Input: part model. Units: mm. Frame: model coordinates. Face numbers are marked on the shaded views. Coordinates: 2 decimals unless noted, no trailing zeros. Loops run counter-clockwise (first coordinate to the right, second up) from the corner with the lowest first, then second, coordinate; pieces in that order, holes last. Notation, with made-up numbers: (70, -38) -> (85, -38) arc R22 ccw to (85, -26) -> close; hole circle Ø2 at (84, -1.5). An arc over 180 degrees is marked (long way). Answer as a JSON object with one key per item and string values.
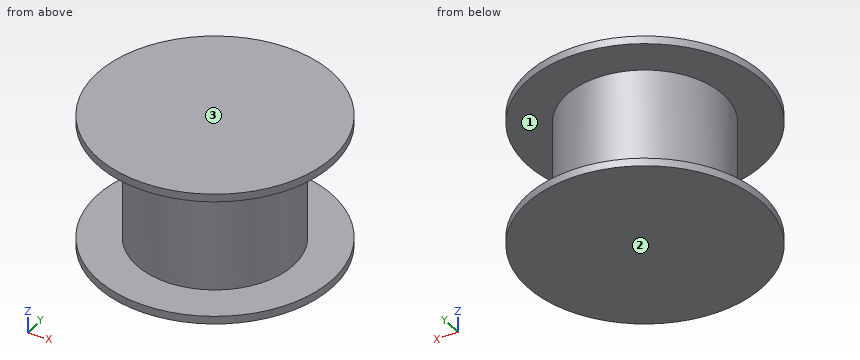
from build123d import *

# Parameters (mm, degrees)
SKETCH1_R           = 10
BOSS_EXTRUDE1_DEPTH = 16
SKETCH2_R           = 15
BOSS_EXTRUDE2_DEPTH = 1
SCALE1_SCALE        = 0.2
SCALE2_SCALE        = 2


with BuildPart() as part:
    # Sketch1 → Boss-Extrude1 (new body)
    with BuildSketch(Plane.XY):
        Circle(SKETCH1_R)
    extrude(amount=BOSS_EXTRUDE1_DEPTH)

    # Sketch2 → Boss-Extrude2 (add)
    with BuildSketch(Plane.XY.offset(16)):
        Circle(SKETCH2_R)
    boss_extrude2 = extrude(amount=-BOSS_EXTRUDE2_DEPTH)

    # Mirror1: Boss-Extrude2 across plane
    add(boss_extrude2.mirror(Plane(origin=(0, 0, 7.5), x_dir=(1, 0, 0), z_dir=(0, 0, -1))))


with BuildPart() as part_1:
    # Scale1: scaled about (0, 0, 7.5)
    add(part.part.scale(SCALE1_SCALE).moved(Location((0, 0, 6))))


with BuildPart() as part_2:
    # Scale2: scaled about (0, 0, 7.5)
    add(part_1.part.scale(SCALE2_SCALE).moved(Location((0, 0, -7.5))))


solid = part_2.part
1. Section query C-C (y = 1.75). Return loops of the section in (x, z).
Reply:
{"outline": "(-5.74, 4.1) -> (5.74, 4.1) -> (5.74, 4.5) -> (3.6, 4.5) -> (3.6, 10.5) -> (5.74, 10.5) -> (5.74, 10.9) -> (-5.74, 10.9) -> (-5.74, 10.5) -> (-3.6, 10.5) -> (-3.6, 4.5) -> (-5.74, 4.5) -> close"}
2. Section query D-D (z = 8). Return loops of the section in (x, y), plus the area to 3 significant figures.
Reply:
{"outline": "circle Ø8 at (0, 0)", "area": "50.3 mm2"}
3. Mould query, pull axis Z, two halves, no side actions, for the marked faces 1, 2 and 3. Classes: pulls with the +Z half, pulls with the -Z half, needs draft (parallel to the pull), parting line crosses it, or undercut.
Reply:
{"face 1": "undercut", "face 2": "pulls with the -Z half", "face 3": "pulls with the +Z half"}
4. Pin query (flat end, axial travel): P1, Ø2, axis at y = 1, z = 8, coming from the -X side; P2, Ø1.5, axis at y = -3, z = 7, coming from the +X side; P3, Ø2, axis at y = 4, z = 6.5, coming from the +X side. Return the tip coordinate at first contact, or that it passes through.
Reply:
{"P1": "stops at x = -4", "P2": "stops at x = 3.31", "P3": "stops at x = 2.65"}
5. Line query: line 1 along Z through (x, y) = (0.5, 4); line 2 along Y through (x, z) = (0, 7.5); line 3 along X through (y, z) = (-3.5, 7.5). Output: solid intervals per line, ascending.
Reply:
{"line 1": "z = 4.1 to 4.5, 10.5 to 10.9", "line 2": "y = -4 to 4", "line 3": "x = -1.94 to 1.94"}
6. Section query B-B (x = 0). Return loops of the section in (y, z), plus the area to 3 significant figures.
Reply:
{"outline": "(-6, 4.1) -> (6, 4.1) -> (6, 4.5) -> (4, 4.5) -> (4, 10.5) -> (6, 10.5) -> (6, 10.9) -> (-6, 10.9) -> (-6, 10.5) -> (-4, 10.5) -> (-4, 4.5) -> (-6, 4.5) -> close", "area": "57.6 mm2"}
7. Section query A-A (y = 5.25). Return loops of the section in (x, z).
Reply:
{"outline": "(-2.9, 4.1) -> (2.9, 4.1) -> (2.9, 4.5) -> (-2.9, 4.5) -> close; (-2.9, 10.5) -> (2.9, 10.5) -> (2.9, 10.9) -> (-2.9, 10.9) -> close"}
